Part print with two shaded views. Sizes in mm from the minimum x, y, z corner. Coordinates: 2 decimals unless noted, no trailing zeros. Loops run counter-clockwise (first coordinate to the right, second up) from the corner with the lowest first, then second, coordinate; pieces in that order, holes last. Notation, with made-up numbers: (14, 35) -> (46, 35) arc R18 cw to (46, 67) -> close; hole circle Ø3 at (-3, 34). An arc over 180 degrees is marked (long way). Write each question's results on one line, items separated by ' | '.
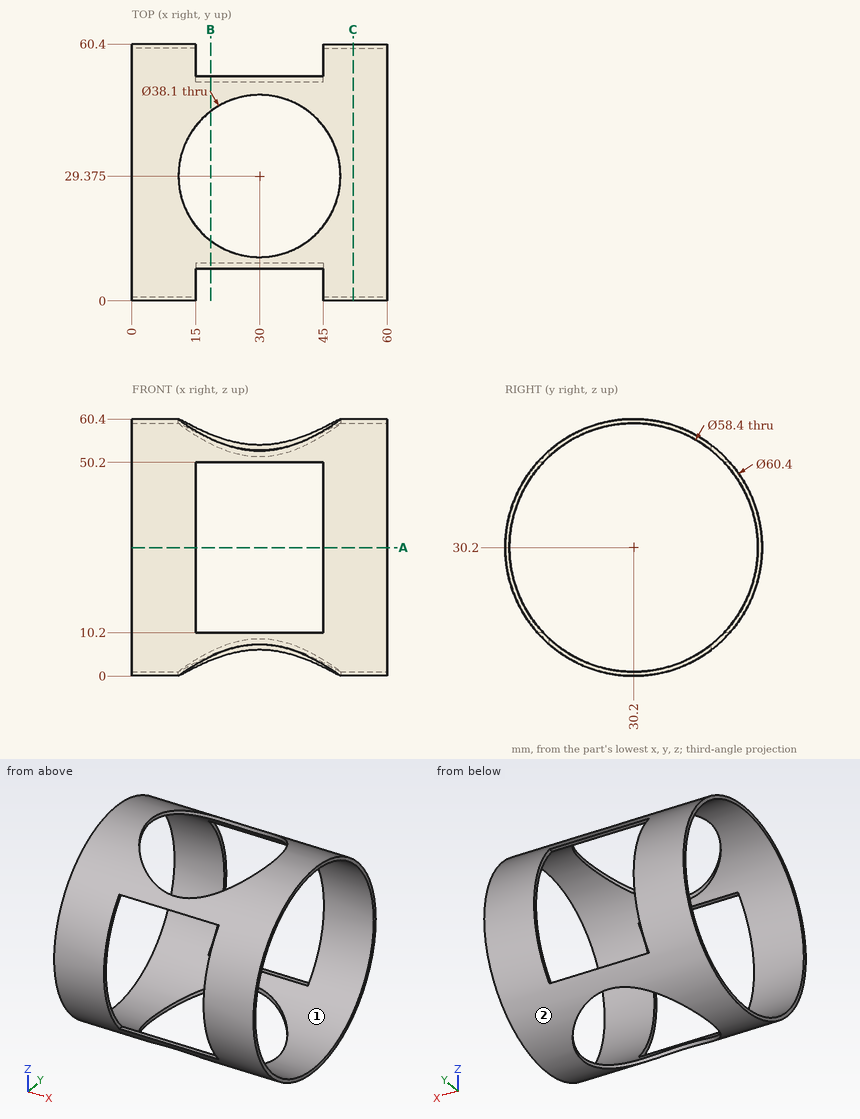
Q1. Cut at B-B on x = 18.5. Write the cut outline in (y, z) (1 decimal).
Results are:
outline: (7.6, 10.2) arc R30.2 ccw to (14.2, 4.6) -> (14.2, 5.8) arc R29.2 cw to (8.9, 10.2) -> close; (7.6, 50.2) -> (8.9, 50.2) arc R29.2 cw to (14.2, 54.6) -> (14.2, 55.8) arc R30.2 ccw to start; (44.6, 3.6) arc R30.2 ccw to (52.8, 10.2) -> (51.5, 10.2) arc R29.2 cw to (44.6, 4.8) -> close; (44.6, 55.6) arc R29.2 cw to (51.5, 50.2) -> (52.8, 50.2) arc R30.2 ccw to (44.6, 56.8) -> close
Q2. Wall check: L1, parallel to Y at x = 55.5, z = 43 (1 decimal); L2, parallel to Z at x = 10, y = 7 (1 decimal); L3, parallel to Z at x = 17, y = 12 (1 decimal). Give the ranges that are in metal, low to high. Write a range as from..to.
Results are:
L1: 2.8..4, 56.4..57.6 | L2: 10.9..12.5, 47.9..49.5 | L3: 6.1..7.4, 53..54.3
Q3. Drop flat-ended pins along their axis: pin 1 (3 mm diameter, centred on x = 6, y = 53, fed in from -Z); pin 2 (1.5 mm diameter, centred on x = 39.5, z = 8.5, fed in from +Y); pin 3 (8 mm diameter, centred on x = 49.5, y = 50, fed in from +Z). Give the stop position or say it passes through.
Results are:
pin 1: z = 8.79 | pin 2: y = 51.95 | pin 3: z = 55.94
Q4. Cut at A-A on z = 30.2. Write the cut outline in (x, y).
Results are:
outline: (0, 0) -> (15, 0) -> (15, 1) -> (0, 1) -> close; (0, 59.4) -> (15, 59.4) -> (15, 60.4) -> (0, 60.4) -> close; (45, 0) -> (60, 0) -> (60, 1) -> (45, 1) -> close; (45, 59.4) -> (60, 59.4) -> (60, 60.4) -> (45, 60.4) -> close
Q5. Cut at C-C on x = 52. Write the cut outline in (y, z).
Results are:
outline: circle Ø60.4 at (30.2, 30.2); hole circle Ø58.4 at (30.2, 30.2)
Q6. Pull direction Z, two halves, no side cores. Call the marked faces 1 and 2: +Z half, -Z half, draft (parallel to the pull), parting line (faces both ways), or undercut.
Results are:
face 1: undercut | face 2: parting line
